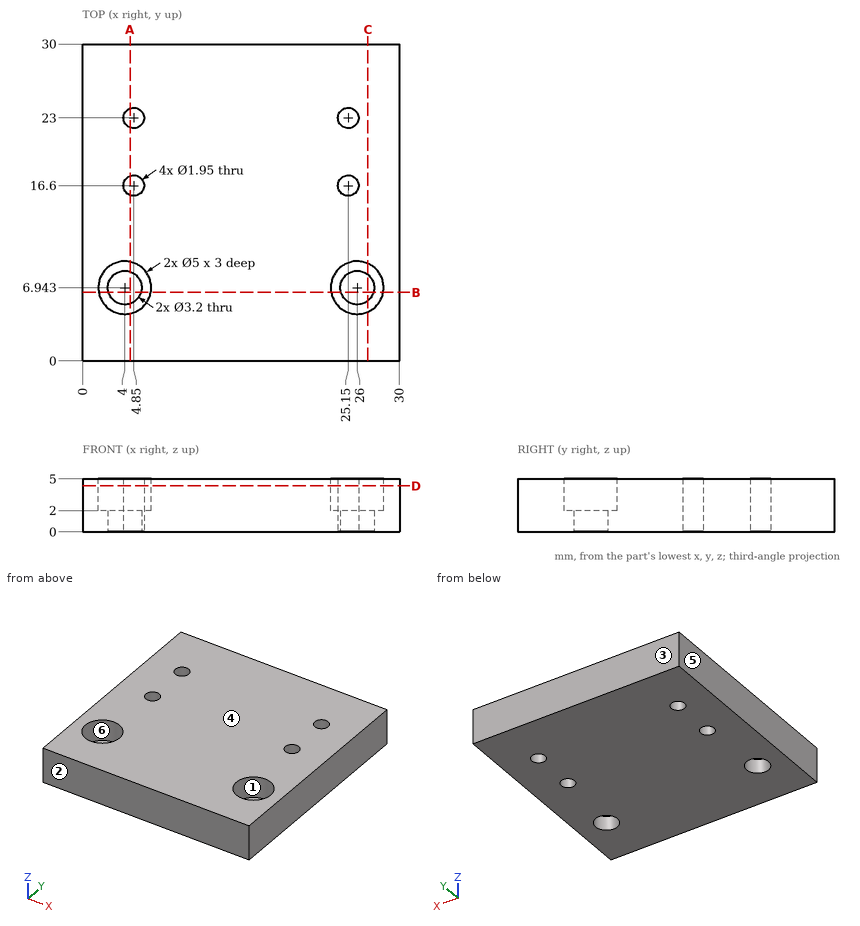
Design review of the part shown in the three views and the two pictorial views. Dimensions are in mm from the part's minimum x, y and z. A direction names the side the tool comes from. Round coordinates to 2 decimals unless told otherwise and drop trailing zeros. Write each loop counter-clockwise with the first axis right and the second up, starting at its lowest first coordinate (ties: lowest second). Pieces come first, ordered by that corner, then holes.
Item 1: The part is to be moulded in two halves that separate along Y. For the marked faces 1, 2, 3 and 4, say which applies: +Y half, -Y half, draft (parallel to the pull), parting line (faces both ways), or undercut.
Item 2: We need section A-A on x = 4.5. Write out the cut boundary in (y, z).
Item 3: For probe 1 along X at (y, z) = (16.75, 4.8); probe 2 along Y at (x, z) = (26, 1.4); probe 3 along Y at (x, z) = (4.85, 1.65) (1 decimal), list the stretches that pass through material, from the lowest coordinate up.
Item 4: We need section D-D on z = 4.35. State how many separate pieces and enclosed holes the cut face has, and give its area (3 significant figures).
Item 5: We need section B-B on y = 6.5. Write out the cut boundary in (x, z), and give its area (3 significant figures).
Item 6: We need section C-C on x = 27. Write out the cut boundary in (y, z).
Item 7: For the marked faces 5 and 6, list the 3-axis set-ups (+Z, -Z, +X, -X, +Y, -Y) from which the entire face can be reached by the end or side of a thin tool; tool diameter is ignored.
Item 8: Clearance check with a flat-ended pin moving along its axis: pin 1 Ø2.5 at (x, y) = (5, 7.5) entering from +Z. State where the tip first meets the part, or that it passes through.
Returned:
1. face 1: undercut
1. face 2: -Y half
1. face 3: +Y half
1. face 4: draft
2. outline: (0, 0) - (5.42, 0) - (5.42, 2) - (4.49, 2) - (4.49, 5) - (0, 5) - close; (8.46, 0) - (15.69, 0) - (15.69, 5) - (9.39, 5) - (9.39, 2) - (8.46, 2) - close; (17.51, 0) - (22.09, 0) - (22.09, 5) - (17.51, 5) - close; (23.91, 0) - (30, 0) - (30, 5) - (23.91, 5) - close
3. probe 1: x = 0 to 3.89, 5.81 to 24.19, 26.11 to 30
3. probe 2: y = 0 to 5.34, 8.54 to 16.12, 17.08 to 22.52, 23.48 to 30
3. probe 3: y = 0 to 5.6, 8.3 to 15.6, 17.6 to 22, 24 to 30
4. separate pieces: 1
4. enclosed holes: 6
4. area: 849 mm2
5. outline: (0, 0) - (2.46, 0) - (2.46, 2) - (1.54, 2) - (1.54, 5) - (0, 5) - close; (5.54, 0) - (24.46, 0) - (24.46, 2) - (23.54, 2) - (23.54, 5) - (6.46, 5) - (6.46, 2) - (5.54, 2) - close; (27.54, 0) - (30, 0) - (30, 5) - (28.46, 5) - (28.46, 2) - (27.54, 2) - close
5. area: 108 mm2
6. outline: (0, 0) - (5.69, 0) - (5.69, 2) - (4.65, 2) - (4.65, 5) - (0, 5) - close; (8.19, 0) - (30, 0) - (30, 5) - (9.23, 5) - (9.23, 2) - (8.19, 2) - close
7. face 5: +Z, -Z, -X, +Y, -Y
7. face 6: +Z
8. pin 1: stops at z = 2
